Check sheet for the modelled part. Datum: model origin and axes. Units: mm. Round coordinates to 2 decimals unless told otherwise and drop trailing zeros. Order: outer loops, then holes, each group sorted by start corner. A loop starts at its lowest first (then second) coordinate and runs counter-clockwise, first axis right, second up.
Q1. Cross-section at B-B on x = -9. Record the cut outline in (y, z) (1 decimal).
Q2. Depth check by flat-ended pin: P1, Ø0.5, axis at y = 26.5, z = 0.5, coming from the +X side; P2, Ø0.8, axis at x = -59.5, z = 0.5, coming from the +Y side; P3, Ø1.3, axis at x = -22.5, z = 1, coming from the +Y side. Enter the tip coordinate at first touch or a pass-through.
Q3. Cross-section at D-D on z = 1.95. Give the number of separate pieces and of enclosed holes in the cut face, then the cut area to 3 significant figures.
Q4. Cross-section at A-A on y = 19.05. Record the cut outline in (x, z) (3 decimals), then the cut area to 3 significant figures.
Q5. Cross-section at C-C on y = 3. Record the cut outline in (x, z) (3 decimals), then the cut area to 3 significant figures.
Q6. Scan lines: probe 1 along Y at (x, z) = (-34.5, 1.95) (1 decimal); probe 2 along X at (y, z) = (-20.5, 0.45); probe 3 along X at (y, z) = (-12.5, 0.15) (3 decimals). Record each from-to range of solid material in increasing order.
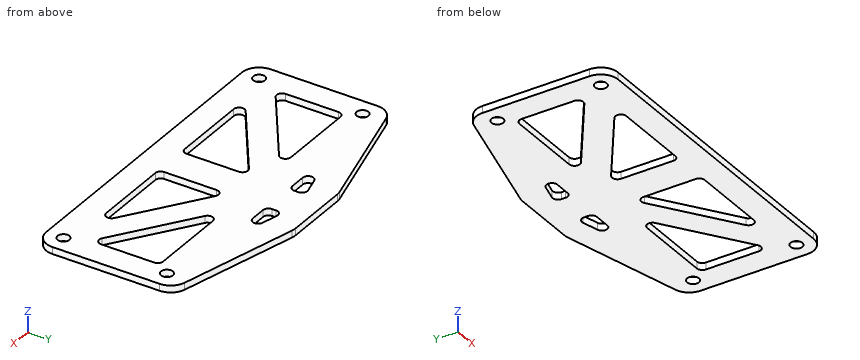
Autodesk Inventor part; units mm, degrees
ref_plane "YZ Plane" through (0, 0, 0) normal (1, 0, 0) x (0, 1, 0)
ref_plane "XZ Plane" through (0, 0, 0) normal (0, 1, 0) x (-1, 0, 0)
ref_plane "XY Plane" through (0, 0, 0) normal (0, 0, 1) x (1, 0, 0)
sketch "Sketch1" plane through (0, 0, 0) normal (0, 0, 1) x (1, 0, 0)
  circle A0 centre (12.7, -19.05) radius 2.1844
  circle A1 centre (12.7, 19.05) radius 2.1844
  circle A2 centre (-98.425, -19.05) radius 2.1844
  circle A3 centre (-98.425, 19.05) radius 2.1844
  line L0 (19.05, -25.4) -> (-104.775, -25.4)
  line L1 (-104.775, -25.4) -> (-104.775, 25.4)
  line L2 (-104.775, 25.4) -> (19.05, 25.4)
  line L3 (19.05, 25.4) -> (19.05, -25.4)
  line L4 (19.05, -25.4) -> (-104.775, 25.4) construction
  line L5 (-104.775, -25.4) -> (19.05, 25.4) construction
  line L6 (19.05, 25.4) -> (-30.1625, 38.1)
  line L7 (-30.1625, 38.1) -> (-55.5625, 38.1)
  line L8 (-55.5625, 38.1) -> (-104.775, 25.4)
  line L9 (-42.8625, 0) -> (-42.8625, 38.1) construction
  point P0 (0, 0)
  dimension "d0" = 6.35
  dimension "d1" = 6.35
  dimension "d2" = 50.8
  dimension "d3" = 6.35
  dimension "d4" = 12.7
  dimension "d6" = 25.4
extrude "Extrusion1" add sketch "Sketch1" along normal blind 2.54
fillet "Fillet1" radius 6.35 6 edges at (19.05, -25.4, 1.27) (19.05, 25.4, 1.27) (-30.1625, 38.1, 1.27) (-55.5625, 38.1, 1.27) (-104.775, 25.4, 1.27) (-104.775, -25.4, 1.27)
sketch "Sketch2" plane through (0, 0, 2.54) normal (0, 0, 1) x (1, 0, 0)
  line L0 (9.525, -11.0599) -> (9.525, 14.2875)
  line L1 (9.525, 14.2875) -> (-27.0917, 14.2875)
  line L2 (-27.0917, 14.2875) -> (9.525, -11.0599)
  line L3 (-12.917, 23.8125) -> (-36.5189, 29.9033)
  line L4 (-36.5189, 29.9033) -> (-36.5189, 23.8125)
  line L5 (-36.5189, 23.8125) -> (-12.917, 23.8125)
  line L6 (-49.2189, 23.8125) -> (-49.2189, 29.9)
  line L7 (-49.2189, 29.9) -> (-72.808, 23.8125)
  line L8 (-72.808, 23.8125) -> (-49.2189, 23.8125)
  line L9 (-0.254, -15.875) -> (-36.5189, 9.2289)
  line L10 (-36.5189, 9.2289) -> (-36.5189, -15.875)
  line L11 (-36.5189, -15.875) -> (-0.254, -15.875)
  line L12 (-49.2189, -15.875) -> (-49.2189, 9.2266)
  line L13 (-49.2189, 9.2266) -> (-85.4731, -15.875)
  line L14 (-85.4731, -15.875) -> (-49.2189, -15.875)
  line L15 (-95.25, -11.0591) -> (-95.25, 14.2875)
  line L16 (-95.25, 14.2875) -> (-58.6421, 14.2875)
  line L17 (-58.6421, 14.2875) -> (-95.25, -11.0591)
  line L18 (-98.425, -25.4) -> (12.7, -25.4)
  line L19 (19.05, -19.05) -> (19.05, 20.4807)
  arc A0 (-29.3819, 37.8986) -> (-30.9686, 38.1) centre (-30.9686, 31.75) ccw
  line L20 (14.2867, 26.6292) -> (-29.3819, 37.8986)
  line L21 (-56.3431, 37.8986) -> (-100.0117, 26.6292)
  circle A1 centre (12.7, 19.05) radius 2.1844
  line L22 (-104.775, 20.4807) -> (-104.775, -19.05)
  circle A2 centre (12.7, -19.05) radius 2.1844
  circle A3 centre (-98.425, -19.05) radius 2.1844
  line L23 (-36.5189, 23.8125) -> (-98.425, -19.05) construction
  line L24 (12.7, -19.05) -> (-49.2189, 23.8125) construction
  point P0 (0, 0)
  point P1 (-30.1689, 38.0494)
  point P2 (-8.7834, 14.2875)
  dimension "d10" = 9.525
  dimension "d11" = 9.525
  dimension "d12" = 12.7
  dimension "d13" = 6.35
  dimension "d14" = 9.525
  dimension "d15" = 9.525
  dimension "d16" = 9.525
  dimension "d17" = 9.525
  dimension "d18" = 4.7625
  dimension "d19" = 9.525
  dimension "d20" = 9.525
  dimension "d21" = 9.525
  dimension "d22" = 4.7625
  dimension "d23" = 4.7625
extrude "Extrusion2" cut sketch "Sketch2" against normal through all contours L2 L1 L0 | L5 L4 L3 | L8 L7 L6 | L11 L10 L9 | L14 L13 L12 | L15 L16 L17
fillet "Fillet2" radius 2 18 edges at (-49.2189, 9.2266, 1.27) (-36.5189, 9.2289, 1.27) (-27.0917, 14.2875, 1.27) (-49.2189, 23.8125, 1.27) (-36.5189, 23.8125, 1.27) (-58.6421, 14.2875, 1.27) (-49.2189, 29.9, 1.27) (-36.5189, 29.9033, 1.27) (-72.808, 23.8125, 1.27) (-12.917, 23.8125, 1.27) (9.525, -11.0599, 1.27) (-0.254, -15.875, 1.27) (9.525, 14.2875, 1.27) (-36.5189, -15.875, 1.27) (-49.2189, -15.875, 1.27) (-95.25, 14.2875, 1.27) (-95.25, -11.0591, 1.27) (-85.4731, -15.875, 1.27)
equation "\"d1\" = d0"
equation "\"d3\" = d0"
properties part number "rangoon"
Results found:
1. outline: (-25.4, 0) - (-15.9, 0) - (-15.9, 2.5) - (-25.4, 2.5) - close; (-9.8, 0) - (1.8, 0) - (1.8, 2.5) - (-9.8, 2.5) - close; (14.3, 0) - (32.6, 0) - (32.6, 2.5) - (14.3, 2.5) - close
2. P1: stops at x = 15.35
2. P2: stops at y = 37.19
2. P3: stops at y = 36.29
3. separate pieces: 1
3. enclosed holes: 10
3. area: 5,270 mm2
4. outline: (-104.775, 0) - (-100.609, 0) - (-100.609, 2.54) - (-104.775, 2.54) - close; (-96.241, 0) - (10.516, 0) - (10.516, 2.54) - (-96.241, 2.54) - close; (14.884, 0) - (19.05, 0) - (19.05, 2.54) - (14.884, 2.54) - close
4. area: 292 mm2
5. outline: (-104.775, 0) - (-95.25, 0) - (-95.25, 2.54) - (-104.775, 2.54) - close; (-74.945, 0) - (-58.212, 0) - (-58.212, 2.54) - (-74.945, 2.54) - close; (-49.219, 0) - (-36.519, 0) - (-36.519, 2.54) - (-49.219, 2.54) - close; (-27.521, 0) - (-10.786, 0) - (-10.786, 2.54) - (-27.521, 2.54) - close; (9.525, 0) - (19.05, 0) - (19.05, 2.54) - (9.525, 2.54) - close
5. area: 166 mm2
6. probe 1: y = -25.4 to -15.9, 7.4 to 23.8, 29.3 to 38.1
6. probe 2: x = -104.61 to -100.06, -96.79 to 11.07, 14.33 to 18.88
6. probe 3: x = -104.775 to -80.523, -49.219 to -36.519, -5.205 to 19.05
